```python
from build123d import *

# Parameters (mm, degrees)
F0_W     = 50
F0_H     = 100
F1_DEPTH = 20
F2_W     = 50
F2_H     = 150
F3_DEPTH = 10
F5_W     = 7
F5_H     = 100
F6_DEPTH = 25


with BuildPart() as f1:
    # F0 (on Top) → F1 (new body)
    with BuildSketch(Plane.XY):
        with Locations((25, 50)):
            Rectangle(F0_W, F0_H)
    extrude(amount=F1_DEPTH)

    # F2 (on Front) → F3 (join)
    with BuildSketch(Plane.XZ):
        with Locations((25, 75)):
            Rectangle(F2_W, F2_H)
    extrude(amount=F3_DEPTH)

    # F5 (on face) → F6 (cut)
    with BuildSketch(Plane.XZ.offset(10)):
        with Locations((26.290544, 82.216139)):
            Rectangle(F5_W, F5_H)
    extrude(amount=-F6_DEPTH, mode=Mode.SUBTRACT)


solid = f1.part
```
CAD build for the part. Positions are in the model's coordinates, mm. A direction names the side the tool comes from. Round coordinates to 2 decimals unless told otherwise and drop trailing zeros. Write each loop counter-clockwise with the first axis right and the second up, starting at its lowest first coordinate (ties: lowest second). Pieces come first, ordered by that corner, then holes. Notation, with made-up numbers: (-24, 50) -> (31, 50) arc R30 cw to (31, 84) -> close; hole circle Ø11 at (-6.5, 14). An arc over 180 degrees is marked (long way). Answer in a Markdown table with one row per item. Add a question column.
Item 1: Drill centre lines: line 1 (Z direction, x = 6.5, y = 94.5); line 2 (Y direction, x = 14.5, z = 28). Where is each one in solid material? Low to high. Write a range as from..to.
Item 2: Saw through at A-A, the plane z = 89.5. Write the cut outline in (x, y).
Item 3: Saw through at C-C, the plane y = 8. Write the cut outline in (x, z), then the cut area to 3 significant figures.
Item 4: Mould opens along X. For faces 4 (the face through (50, 33, 19)), 5 (the face through (19, 0, 86)), 6 (the face through (26, -5, 32.216)) say: pulls with the +X half, pulls with the -X half, needs draft (parallel to the pull), parting line crosses it, or undercut.
Item 5: Which spindle directions (+Z, -Z, +X, -X, +Y, -Y) get a long thin tool onto all of the face, cutting with end or side? Do faces 1 (the face through (19, -10, 76)), 2 (the face through (26, -5, 132.216)), 3 (the face through (25, 51, 20)). Say none if no direction does.
Item 6: Saw through at B-B, the plane x = 40. Write the cut outline in (y, z), then the cut area to 3 significant figures.
Item 7: Drop flat-ended pins along their axis: pin 1 Ø6 at (x, y) = (9, 11) entering from +Z; pin 2 Ø15 at (x, z) = (30, 63) entering from +Y. Give the stop position or say it passes through.
Findings below:
| question | item | result |
|---|---|---|
| 1 | line 1 | z = 0..20 |
| 1 | line 2 | y = -10..0 |
| 2 | outline | (0, -10) -> (22.79, -10) -> (22.79, 0) -> (0, 0) -> close; (29.79, -10) -> (50, -10) -> (50, 0) -> (29.79, 0) -> close |
| 3 | outline | (0, 0) -> (50, 0) -> (50, 20) -> (0, 20) -> close |
| 3 | area | 1,000 mm^2 |
| 4 | face 4 | pulls with the +X half |
| 4 | face 5 | needs draft |
| 4 | face 6 | undercut |
| 5 | face 1 | +Z, -Z, +X, -X, -Y |
| 5 | face 2 | +Y, -Y |
| 5 | face 3 | +Z, +X, -X, +Y |
| 6 | outline | (-10, 0) -> (100, 0) -> (100, 20) -> (0, 20) -> (0, 150) -> (-10, 150) -> close |
| 6 | area | 3,500 mm^2 |
| 7 | pin 1 | stops at z = 20 |
| 7 | pin 2 | stops at y = 0 |
